Geometry check sheet. Reference: the model listing, model coordinates, mm. Coordinates: 2 decimals unless noted, no trailing zeros. Loops run counter-clockwise (first coordinate to the right, second up) from the corner with the lowest first, then second, coordinate; pieces in that order, holes last. Notation, with made-up numbers: (-34.75, -38.5) -> (3.25, -38.5) arc R29 cw to (3.25, -8.5) -> close; hole circle Ø11 at (32, 23). An arc over 180 degrees is marked (long way). Answer as a JSON object with one key per item and string values.
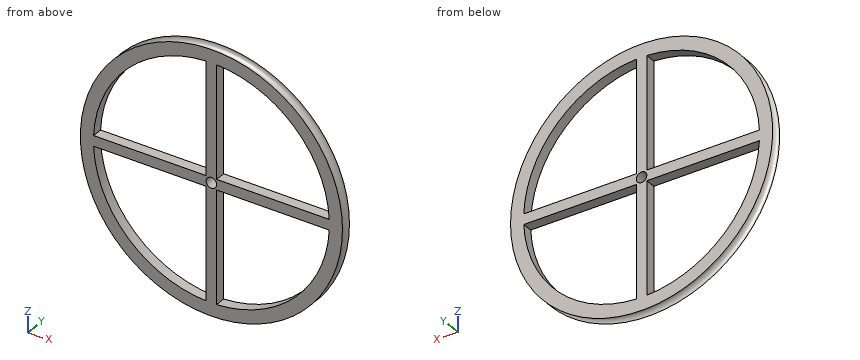
from build123d import *

# Parameters (mm, degrees)
F2_R     = 1
F3_DEPTH = 25
F5_DEPTH = 25


with BuildPart() as f1:
    # F0 (on Top) → F1 (revolve)
    with BuildSketch(Plane.XY):
        with BuildLine():
            Line((25, 0), (0, 0))
            Line((0, 0), (0, -2))
            Line((0, -2), (25, -2))
            ThreePointArc((25, -2), (24, -1), (25, 0))
        make_face()
    revolve(axis=Axis((0, -1, 0), (0, -1, 0)))

    # F2 (on face) → F3 (cut)
    with BuildSketch(Plane.XZ.offset(2)):
        Circle(F2_R)
    extrude(amount=-F3_DEPTH, mode=Mode.SUBTRACT)

    # F4 (on face) → F5 (cut)
    with BuildSketch(Plane.XZ.offset(2)):
        with BuildLine():
            Line((-1, 1), (-1, 22.477766793))
            ThreePointArc((-1, 22.477766793), (-15.9099025767, 15.9099025767), (-22.477766793, 1))
            Line((-22.477766793, 1), (-1, 1))
        make_face()
        with BuildLine():
            ThreePointArc((-22.477766793, -1), (-15.9099025767, -15.9099025767), (-1, -22.477766793))
            Line((-1, -22.477766793), (-1, -1))
            Line((-1, -1), (-22.477766793, -1))
        make_face()
        with BuildLine():
            ThreePointArc((1, -22.477766793), (15.9099025767, -15.9099025767), (22.477766793, -1))
            Line((22.477766793, -1), (1, -1))
            Line((1, -1), (1, -22.477766793))
        make_face()
        with BuildLine():
            Line((1, 1), (22.477766793, 1))
            ThreePointArc((22.477766793, 1), (15.9099025767, 15.9099025767), (1, 22.477766793))
            Line((1, 22.477766793), (1, 1))
        make_face()
    extrude(amount=-F5_DEPTH, mode=Mode.SUBTRACT)


solid = f1.part
1. Depth check by flat-ended pin: P1, Ø0.6, axis at x = 7.5, y = -1, coming from the +Z side; P2, Ø0.6, axis at x = 8, y = -1, coming from the -Z side; P3, Ø3, axis at x = 0, z = 0, coming from the -Y side. Enter the tip coordinate at first touch or a pass-through.
Evaluation:
{"P1": "stops at z = 22.89", "P2": "stops at z = -22.73", "P3": "stops at y = -2"}
2. Section check B-B, the plane z = 0. Record the boundary of the cut face in (x, y).
Evaluation:
{"outline": "(-25, -2) -> (-1, -2) -> (-1, 0) -> (-25, 0) arc R1 cw to start; (1, -2) -> (25, -2) arc R1 cw to (25, 0) -> (1, 0) -> close"}
3. Section check A-A, the plane x = 0. Record the boundary of the cut face in (y, z), then the cut area to 3 significant figures.
Evaluation:
{"outline": "(-2, -25) arc R1 cw to (0, -25) -> (0, -1) -> (-2, -1) -> close; (-2, 1) -> (0, 1) -> (0, 25) arc R1 cw to (-2, 25) -> close", "area": "92.9 mm^2"}
4. Section check D-D, the plane z = -11. State how many separate pieces and enclosed holes the cut face has, then the cut area to 3 significant figures.
Evaluation:
{"separate pieces": "3", "enclosed holes": "0", "area": "11.8 mm^2"}
5. Thickness scan on probe 1 along Z at (x, y) = (-7, -1.6); probe 2 along X at (y, z) = (-1.45, 14.5); probe 3 along X at (y, z) = (-1.4, 6). Record the ranges inside material, lowest first. Write a range as from..to.
Evaluation:
{"probe 1": "z = -23.17..-21.38, -1..1, 21.38..23.17", "probe 2": "x = -19.26..-17.2, -1..1, 17.2..19.26", "probe 3": "x = -23.32..-21.69, -1..1, 21.69..23.32"}
6. Section check C-C, the plane y = -0.45. Record the boundary of the cut face in (x, z).
Evaluation:
{"outline": "circle Ø48.33 at (0, 0); hole (-22.48, -1) arc R22.5 ccw to (-1, -22.48) -> (-1, -1) -> close; hole (-22.48, 1) -> (-1, 1) -> (-1, 22.48) arc R22.5 ccw to start; hole circle Ø2 at (0, 0); hole (1, -22.48) arc R22.5 ccw to (22.48, -1) -> (1, -1) -> close; hole (1, 1) -> (22.48, 1) arc R22.5 ccw to (1, 22.48) -> close"}
